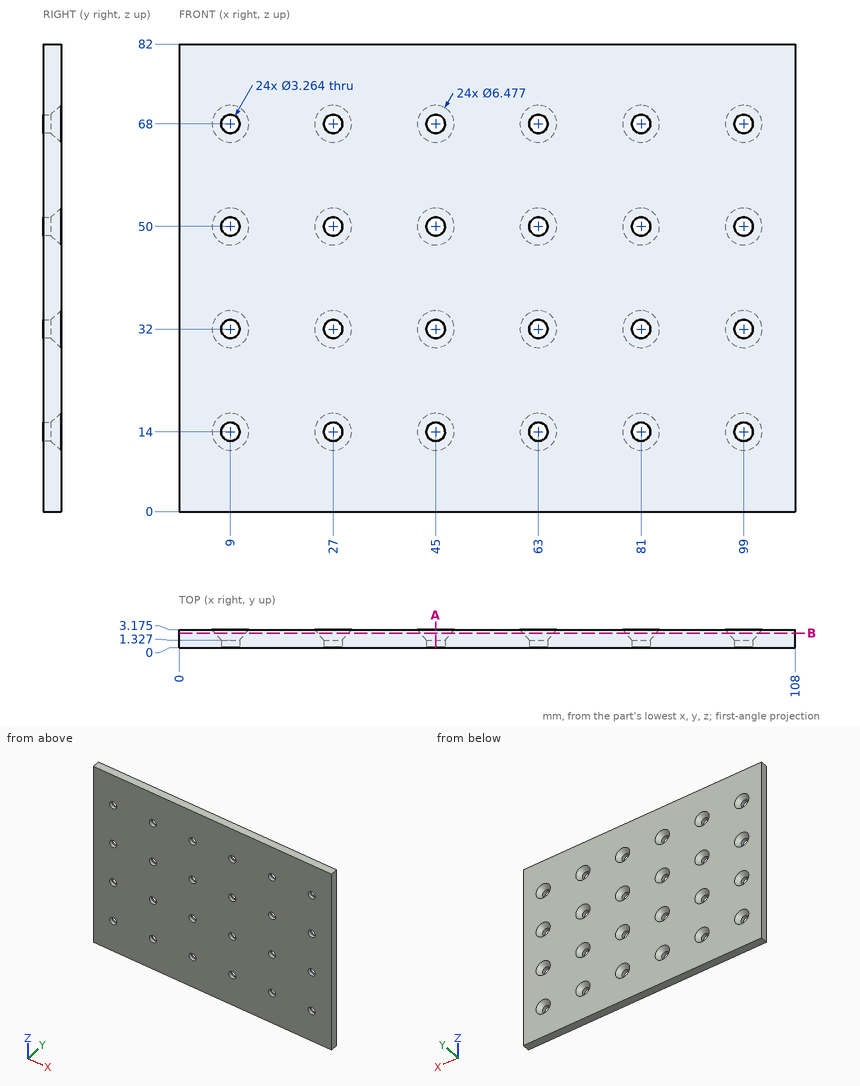
Verification items for this drawing (mm, ordinates from the low corner). Coordinates: 2 decimals unless noted, no trailing zeros. Loops run counter-clockwise (first coordinate to the right, second up) from the corner with the lowest first, then second, coordinate; pieces in that order, holes last.
Item 1: Sectioned sample at B-B, the plane y = 2.55. Count the separate pieces of the cut face and the enclosed holes in it, then the cut area to 3 significant figures.
Item 2: Go/stop test with flat-tipped pins: pin 1 Ø4 at (x, z) = (9, 32) entering from +Y; pin 2 Ø3 at (x, z) = (81, 68) entering from -Y. Record where each tip stops, or that it passes through.
Item 3: Thickness scan on line 1 (Z direction, x = 99, y = 0.65); line 2 (Z direction, x = 82.5, y = 1.9); line 3 (Y direction, x = 25, z = 30.5) (1 decimal). Record the ranges inside material, lowest first.
Item 4: Sectioned sample at A-A, the plane x = 45. Record the boundary of the cut face in (y, z) (1 decimal).
Check result:
1. separate pieces: 1
1. enclosed holes: 24
1. area: 8,310 mm2
2. pin 1: stops at y = 1.75
2. pin 2: passes through
3. line 1: z = 0 to 12.37, 15.63 to 30.37, 33.63 to 48.37, 51.63 to 66.37, 69.63 to 82
3. line 2: z = 0 to 12.49, 15.51 to 30.49, 33.51 to 48.49, 51.51 to 66.49, 69.51 to 82
3. line 3: y = 0 to 2.3
4. outline: (0, 0) - (3.2, 0) - (3.2, 10.8) - (1.3, 12.4) - (0, 12.4) - close; (0, 15.6) - (1.3, 15.6) - (3.2, 17.2) - (3.2, 28.8) - (1.3, 30.4) - (0, 30.4) - close; (0, 33.6) - (1.3, 33.6) - (3.2, 35.2) - (3.2, 46.8) - (1.3, 48.4) - (0, 48.4) - close; (0, 51.6) - (1.3, 51.6) - (3.2, 53.2) - (3.2, 64.8) - (1.3, 66.4) - (0, 66.4) - close; (0, 69.6) - (1.3, 69.6) - (3.2, 71.2) - (3.2, 82) - (0, 82) - close
